Source: CAD feature listing. Evaluate the final solid. Frame: model axes, mm. A direction names the side the tool comes from. Round coordinates to 2 decimals unless told otherwise and drop trailing zeros. Write each loop counter-clockwise with the first axis right and the second up, starting at its lowest first coordinate (ties: lowest second). Pieces come first, ordered by that corner, then holes. Notation, with made-up numbers: (0.25, 5) -> (39.25, 5) arc R21 ccw to (39.25, 32) -> close; hole circle Ø6 at (87, 82). An arc over 180 degrees is marked (long way). Put each result on its own line as item: value.
```python
from build123d import *

# Parameters (mm, degrees)
ESQUISSE1_R        = 2.15
BOSS_EXTRU_1_DEPTH = 50


with BuildPart() as part:
    # Esquisse1 → Boss.-Extru.1 (new body)
    with BuildSketch(Plane(origin=(0, 0, 0), x_dir=(-1, 0, 0), z_dir=(0, 0, -1))):
        with BuildLine():
            Line((-17.999994246, 0), (-1.999994246, 0))
            ThreePointArc((-1.999994246, 0), (-0.585780683, 0.585786438), (5.754e-06, 2))
            Line((5.754e-06, 2), (5.754e-06, 6.699994246))
            ThreePointArc((5.754e-06, 6.699994246), (-0.234308821, 7.265679671), (-0.799994246, 7.499994246))
            Line((-0.799994246, 7.499994246), (-1.499994246, 7.499994246))
            ThreePointArc((-1.499994246, 7.499994246), (-1.71212628, 7.41212628), (-1.799994246, 7.199994246))
            Line((-1.799994246, 7.199994246), (-1.799994246, 5.081575939))
            ThreePointArc((-1.799994246, 5.081575939), (-2.31333985, 4.313299949), (-3.21958317, 4.493562953))
            Line((-3.21958317, 4.493562953), (-5.471314589, 6.745294373))
            ThreePointArc((-5.471314589, 6.745294373), (-6.121632843, 7.718564419), (-6.349994246, 8.866614716))
            Line((-6.349994246, 8.866614716), (-6.349994246, 11.133385284))
            ThreePointArc((-6.349994246, 11.133385284), (-6.121632843, 12.281435581), (-5.471314589, 13.254705627))
            Line((-5.471314589, 13.254705627), (-3.21958317, 15.506437047))
            ThreePointArc((-3.21958317, 15.506437047), (-2.31333985, 15.686700051), (-1.799994246, 14.918424061))
            Line((-1.799994246, 14.918424061), (-1.799994246, 12.799994246))
            ThreePointArc((-1.799994246, 12.799994246), (-1.71212628, 12.587862211), (-1.499994246, 12.499994246))
            Line((-1.499994246, 12.499994246), (-0.799994246, 12.499994246))
            ThreePointArc((-0.799994246, 12.499994246), (-0.234308821, 12.734308821), (5.754e-06, 13.299994246))
            Line((5.754e-06, 13.299994246), (5.754e-06, 18))
            ThreePointArc((5.754e-06, 18), (-0.585780683, 19.414213562), (-1.999994246, 20))
            Line((-1.999994246, 20), (-6.699994246, 20))
            ThreePointArc((-6.699994246, 20), (-7.265679671, 19.765685425), (-7.499994246, 19.2))
            Line((-7.499994246, 19.2), (-7.499994246, 18.5))
            ThreePointArc((-7.499994246, 18.5), (-7.41212628, 18.287867966), (-7.199994246, 18.2))
            Line((-7.199994246, 18.2), (-5.081570185, 18.2))
            ThreePointArc((-5.081570185, 18.2), (-4.313294195, 17.686654396), (-4.493557199, 16.780411076))
            Line((-4.493557199, 16.780411076), (-6.745288618, 14.528679656))
            ThreePointArc((-6.745288618, 14.528679656), (-7.718558665, 13.878361402), (-8.866608962, 13.65))
            Line((-8.866608962, 13.65), (-11.13337953, 13.65))
            ThreePointArc((-11.13337953, 13.65), (-12.281429827, 13.878361402), (-13.254699873, 14.528679656))
            Line((-13.254699873, 14.528679656), (-15.506431292, 16.780411076))
            ThreePointArc((-15.506431292, 16.780411076), (-15.686694297, 17.686654396), (-14.918418307, 18.2))
            Line((-14.918418307, 18.2), (-12.799994246, 18.2))
            ThreePointArc((-12.799994246, 18.2), (-12.587862211, 18.287867966), (-12.499994246, 18.5))
            Line((-12.499994246, 18.5), (-12.499994246, 19.2))
            ThreePointArc((-12.499994246, 19.2), (-12.734308821, 19.765685425), (-13.299994246, 20))
            Line((-13.299994246, 20), (-17.999994246, 20))
            ThreePointArc((-17.999994246, 20), (-19.414207808, 19.414213562), (-19.999994246, 18))
            Line((-19.999994246, 18), (-19.999994246, 2))
            ThreePointArc((-19.999994246, 2), (-19.414207808, 0.585786438), (-17.999994246, 0))
        make_face()
        with Locations(Location((-10, 10, 0), (0, 0, 180))):
            Circle(ESQUISSE1_R, mode=Mode.SUBTRACT)
        with BuildLine():
            Line((-16.778984489, 15.506192283), (-14.528680848, 13.255888642))
            ThreePointArc((-14.528680848, 13.255888642), (-13.878362594, 12.282618596), (-13.650001192, 11.134568298))
            Line((-13.650001192, 11.134568298), (-13.650001192, 8.865430016))
            ThreePointArc((-13.650001192, 8.865430016), (-13.878362594, 7.717379719), (-14.528680848, 6.744109673))
            Line((-14.528680848, 6.744109673), (-16.778991435, 4.493799086))
            ThreePointArc((-16.778991435, 4.493799086), (-17.686141031, 4.313355812), (-18.2, 5.082400105))
            Line((-18.2, 5.082400105), (-18.2, 7.199994246))
            ThreePointArc((-18.2, 7.199994246), (-18.287867966, 7.41212628), (-18.5, 7.499994246))
            Line((-18.5, 7.499994246), (-19, 7.499994246))
            ThreePointArc((-19, 7.499994246), (-19.212132034, 7.587862211), (-19.3, 7.799994246))
            Line((-19.3, 7.799994246), (-19.3, 12.199994246))
            ThreePointArc((-19.3, 12.199994246), (-19.212132034, 12.41212628), (-19, 12.499994246))
            Line((-19, 12.499994246), (-18.5, 12.499994246))
            ThreePointArc((-18.5, 12.499994246), (-18.287867966, 12.587862211), (-18.2, 12.799994246))
            Line((-18.2, 12.799994246), (-18.2, 14.917588386))
            ThreePointArc((-18.2, 14.917588386), (-17.68613852, 15.686636439), (-16.778984489, 15.506192283))
        make_face(mode=Mode.SUBTRACT)
        with BuildLine():
            Line((-15.506192283, 3.221015511), (-13.25588745, 5.471320344))
            ThreePointArc((-13.25588745, 5.471320344), (-12.282617404, 6.121638598), (-11.134567107, 6.35))
            Line((-11.134567107, 6.35), (-8.865432893, 6.35))
            ThreePointArc((-8.865432893, 6.35), (-7.717382596, 6.121638598), (-6.74411255, 5.471320344))
            Line((-6.74411255, 5.471320344), (-4.493800771, 3.221008565))
            ThreePointArc((-4.493800771, 3.221008565), (-4.313357497, 2.313858969), (-5.082401791, 1.8))
            Line((-5.082401791, 1.8), (-7.199994246, 1.8))
            ThreePointArc((-7.199994246, 1.8), (-7.41212628, 1.712132034), (-7.499994246, 1.5))
            Line((-7.499994246, 1.5), (-7.499994246, 1))
            ThreePointArc((-7.499994246, 1), (-7.587862211, 0.787867966), (-7.799994246, 0.7))
            Line((-7.799994246, 0.7), (-12.199994246, 0.7))
            ThreePointArc((-12.199994246, 0.7), (-12.41212628, 0.787867966), (-12.499994246, 1))
            Line((-12.499994246, 1), (-12.499994246, 1.5))
            ThreePointArc((-12.499994246, 1.5), (-12.587862211, 1.712132034), (-12.799994246, 1.8))
            Line((-12.799994246, 1.8), (-14.917588386, 1.8))
            ThreePointArc((-14.917588386, 1.8), (-15.686636439, 2.31386148), (-15.506192283, 3.221015511))
        make_face(mode=Mode.SUBTRACT)
    extrude(amount=-BOSS_EXTRU_1_DEPTH)


solid = part.part
```
Q1. Pin query (flat end, axial travel): pin 1 (1 mm diameter, centred on x = 15, z = 22, fed in from -Y); pin 2 (1.3 mm diameter, centred on y = 10, z = 29.5, fed in from -X); pin 3 (0.6 mm diameter, centred on y = 1, z = 22, fed in from +X); pin 4 (0.6 mm diameter, centred on y = 1.5, z = 36.5, fed in from -X). Return the tip coordinate at first contact, or that it passes through.
Ans:
pin 1: stops at y = 0
pin 2: stops at x = 6.35
pin 3: stops at x = 19.87
pin 4: stops at x = 0.01
Q2. Material intervals for line 1 (X direction, y = 10, z = 26); line 2 (Y direction, x = 10, z = 18); line 3 (Y direction, x = 2.5, z = 23), sorted ascending. Write a range as [from, to].
Ans:
line 1: x = [6.35, 7.85], [12.15, 13.65], [19.3, 20]
line 2: y = [0, 0.7], [6.35, 7.85], [12.15, 13.65]
line 3: y = [0, 4.26], [15.74, 20]
Q3. Draft query along Y for faces 3 (the flat face through (10, 13.65, 25)), 4 (the cylindrical face through (0.6, 0.57, 24.65)), 5 (the flat face through (12.4, 10.1, 0)), 6 (the cylindrical face through (13.872, 7.733, 24.65)). Return one class per face: +Y half, -Y half, draft (parallel to the pull), parting line (faces both ways), or undercut.
Ans:
face 3: +Y half
face 4: -Y half
face 5: draft
face 6: undercut
Q4. Cut plane C-C on z = 37. Give the number of separate pieces and of enclosed holes in the cut face, and give its area (3 significant figures).
Ans:
separate pieces: 1
enclosed holes: 3
area: 191 mm^2
Q5. Reachability of faces 1 (the cylindrical face through (19.43, 0.6, 24.65)), 2 (the flat face through (1.8, 6, 25)) from +Z, -Z, +X, -X, +Y, -Y: full face, straight path, thin tool, end or side. Return the list, or none.
Ans:
face 1: +Z, -Z, +X, -Y
face 2: +Z, -Z
Q6. Cut plane B-B on x = 2.75. Output: boundary loops of the cut face in (y, z), and give its area (3 significant figures).
Ans:
outline: (0, 0) -> (4.26, 0) -> (4.26, 50) -> (0, 50) -> close; (15.74, 0) -> (20, 0) -> (20, 50) -> (15.74, 50) -> close
area: 426 mm^2
Q7. Cut plane A-A on x = 10. Output: boundary loops of the cut face in (y, z), and give its area (3 significant figures).
Ans:
outline: (0, 0) -> (0.7, 0) -> (0.7, 50) -> (0, 50) -> close; (6.35, 0) -> (7.85, 0) -> (7.85, 50) -> (6.35, 50) -> close; (12.15, 0) -> (13.65, 0) -> (13.65, 50) -> (12.15, 50) -> close
area: 185 mm^2
